Read the model definition and answer for the solid it produces. Units are mm, in the model's axes. Coordinates: 2 decimals unless noted, no trailing zeros. Order: outer loops, then holes, each group sorted by start corner. A loop starts at its lowest first (then second) coordinate and runs counter-clockwise, first axis right, second up.
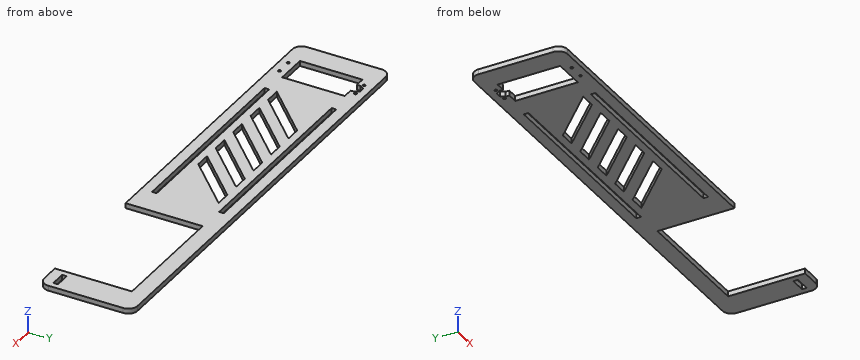
Autodesk Inventor part; units mm, degrees
ref_plane "YZ Plane" through (0, 0, 0) normal (1, 0, 0) x (0, 1, 0)
ref_plane "XZ Plane" through (0, 0, 0) normal (0, 1, 0) x (-1, 0, 0)
ref_plane "XY Plane" through (0, 0, 0) normal (0, 0, 1) x (1, 0, 0)
sketch "Sketch7" plane through (0, 0, 0) normal (0, 0, 1) x (1, 0, 0)
  line L0 (296.3, 0) -> (296.3, 60.7)
  line L1 (296.3, 60.7) -> (0, 60.7)
  line L2 (0, 60.7) -> (0, 0)
  line L3 (50.3, 10) -> (179.25, 10)
  line L4 (179.25, 10) -> (179.25, 7)
  line L5 (179.25, 7) -> (50.3, 7)
  line L6 (50.3, 7) -> (50.3, 10)
  line L7 (15, 50.75) -> (35.3, 50.75)
  line L8 (35.3, 50.75) -> (35.3, 9.95)
  line L9 (35.3, 9.95) -> (15, 9.95)
  line L10 (15, 9.95) -> (15, 50.75)
  line L11 (50.3, 50.7) -> (179.25, 50.7)
  line L12 (179.25, 50.7) -> (179.25, 53.7)
  line L13 (179.25, 53.7) -> (50.3, 53.7)
  line L14 (50.3, 53.7) -> (50.3, 50.7)
  line L15 (0, 0) -> (197.25, 0)
  line L16 (197.25, 0) -> (197.25, 50.2)
  line L17 (197.25, 50.2) -> (278.3, 50.2)
  line L18 (278.3, 50.2) -> (278.3, 0)
  line L19 (278.3, 0) -> (296.3, 0)
  line L20 (282.3, 10) -> (292.3, 10)
  line L21 (292.3, 10) -> (292.3, 7)
  line L22 (292.3, 7) -> (282.3, 7)
  line L23 (282.3, 7) -> (282.3, 10)
  point P0 (50.3, 52.2)
  point P1 (50.3, 8.5)
  dimension "d154" = 128.95
  dimension "d159" = 3
  dimension "d161" = 40.8
  dimension "d162" = 20.3
  dimension "d163" = 15
  dimension "d168" = 7
  dimension "d224" = 40.7
  dimension "d225" = 15
  dimension "d232" = 60.7
  dimension "d233" = 7
  dimension "d234" = 18
  dimension "d235" = 81.05
  dimension "d236" = 9.95
  dimension "d237" = 10.5
  dimension "d239" = 18
  dimension "d240" = 4
  dimension "d247" = 10
extrude "Extrusion7" add sketch "Sketch7" along normal blind 3.3 contours L19 L18 L17 L16 L15 L2 L1 L0 | L20 L21 L22 L23
fillet "Fillet1" radius 6 4 edges at (0, 60.7, 1.65) (0, 0, 1.65) (296.3, 60.7, 1.65) (296.3, 0, 1.65)
sketch "Sketch9" plane through (0, 0, 3.3) normal (0, 0, 1) x (1, 0, 0)
  arc A0 (290.3, 0) -> (296.3, 6) centre (290.3, 6) ccw
  line L0 (296.3, 6) -> (296.3, 54.7)
  arc A1 (296.3, 54.7) -> (290.3, 60.7) centre (290.3, 54.7) ccw
  line L1 (290.3, 60.7) -> (6, 60.7)
  arc A2 (6, 60.7) -> (0, 54.7) centre (6, 54.7) ccw
  line L2 (0, 54.7) -> (0, 6)
  arc A3 (0, 6) -> (6, 0) centre (6, 6) ccw
  line L3 (35.3, 50.75) -> (35.3, 9.95)
  line L4 (35.3, 9.95) -> (15, 9.95)
  line L5 (15, 9.95) -> (15, 50.75)
  line L6 (15, 50.75) -> (35.3, 50.75)
  line L7 (50.3, 50.7) -> (50.3, 53.7)
  line L8 (50.3, 53.7) -> (179.25, 53.7)
  line L9 (179.25, 53.7) -> (179.25, 50.7)
  line L10 (179.25, 50.7) -> (50.3, 50.7)
  line L11 (179.25, 10) -> (179.25, 7)
  line L12 (179.25, 7) -> (50.3, 7)
  line L13 (50.3, 7) -> (50.3, 10)
  line L14 (50.3, 10) -> (179.25, 10)
  line L15 (50.3, 15) -> (81, 45.7)
  line L16 (81, 45.7) -> (91, 45.7)
  line L17 (91, 45.7) -> (60.3, 15)
  line L18 (60.3, 15) -> (50.3, 15)
  line L19 (6, 0) -> (197.25, 0)
  line L20 (197.25, 0) -> (197.25, 50.2)
  line L21 (197.25, 50.2) -> (278.3, 50.2)
  line L22 (278.3, 50.2) -> (278.3, 0)
  line L23 (278.3, 0) -> (290.3, 0)
  point P0 (0, 0)
  dimension "d172" = 45
  dimension "d173" = 10
  dimension "d175" = 5
  dimension "d182" = 5
extrude "Extrusion8" cut sketch "Sketch9" against normal blind 3.3 contours L15 L16 L17 L18
sketch "Sketch10" plane through (0, 0, 3.3) normal (0, 0, 1) x (1, 0, 0)
  line L0 (15, 9.95) -> (15, 50.75)
  line L1 (15, 50.75) -> (35.3, 50.75)
  line L2 (35.3, 50.75) -> (35.3, 9.95)
  line L3 (35.3, 9.95) -> (15, 9.95)
  circle A0 centre (20, 54.7) radius 0.85
  circle A1 centre (30, 54.7) radius 0.85
  circle A2 centre (20, 5.2) radius 0.85
  circle A3 centre (30, 5.2) radius 0.85
  point P0 (0, 0)
  dimension "d183" = 1.7
  dimension "d184" = 5
  dimension "d185" = 10
  dimension "d186" = 5
  dimension "d187" = 10
  dimension "d188" = 3.95
  dimension "d189" = 4.75
extrude "Extrusion9" cut sketch "Sketch10" against normal blind 10 contours A0 | A1 | A2 | A3
sketch "Sketch11" plane through (0, 0, 3.3) normal (0, 0, 1) x (1, 0, 0)
  line L0 (15, 50.75) -> (35.3, 50.75)
  line L1 (21.4, 55.85) -> (28.6, 55.85) construction
  line L2 (28.6, 55.85) -> (28.6, 50.75) construction
  line L3 (28.6, 50.75) -> (21.4, 50.75)
  line L4 (21.4, 50.75) -> (21.4, 55.85) construction
  line L5 (15, 9.95) -> (15, 50.75)
  line L6 (35.3, 50.75) -> (35.3, 9.95)
  line L7 (259.7, 10) -> (259.7, 50.8)
  line L8 (21.4, 53.25) -> (23.2205, 55.85)
  line L9 (26.7795, 55.85) -> (28.6, 53.25)
  line L10 (21.4, 50.75) -> (21.4, 53.25)
  line L11 (23.2205, 55.85) -> (26.7795, 55.85)
  line L12 (28.6, 53.25) -> (28.6, 50.75)
  point P0 (0, 0)
  dimension "d203" = 6.4
  dimension "d205" = 5.1
  dimension "d206" = 7.2
  dimension "d215" = 35
  dimension "d216" = 2.5
  dimension "d217" = 35
extrude "Extrusion10" cut sketch "Sketch11" against normal blind 10
sketch "Sketch13" plane through (0, 0, 3.3) normal (0, 0, 1) x (1, 0, 0)
  line L0 (282.3, 10) -> (292.3, 10)
  line L1 (292.3, 10) -> (292.3, 7)
  line L2 (292.3, 7) -> (282.3, 7)
  line L3 (282.3, 7) -> (282.3, 10)
  point P0 (0, 0)
extrude "Extrusion11" cut sketch "Sketch13" against normal up to surface (3.3 mm away)
pattern_linear "Rectangular Pattern2" count 5 spacing 20 along (1, 0, 0) of "Extrusion8"
equation "\"base_servo\" = 20"
equation "\"altura_servo\" = 40"
equation "\"agujero_servo\" = 2"
equation "\"distancia_agujero_servo\" = 4.75"
equation "\"largo_base\" = 200"
properties part number "Cuerpo - LateralPrueba"
Q1. This flat-tipped pin is pushed along its axis until it touches: P1, Ø1.4, axis at x = 20, y = 5.2, coming from the +Z side. Where does it stop, or does it pass through?
Q2. The part is cut by section B-B, the plane y = 18. State how many separate pieces and enclosed holes the cut face has, then the cut area to 3 significant figures.
Q3. Straight lines are drawn through the part: L1, parallel to X at y = 11, z = 0.45; L2, parallel to Y at x = 30, z = 0.8; L3, parallel to Y at x = 139.5, z = 2.55. For each, find the intervals that lie inside material, in ascending order.
Q4. The part is cut by section D-D, the plane x = 237. Determine the outline of the cut face in (y, z), then the cut area to 4 significant figures.
Q5. The part is cut by section A-A, the plane x = 137. Determine the outline of the cut face in (y, z).
Computed values:
1. P1: passes through
2. separate pieces: 8
2. enclosed holes: 0
2. area: 478 mm2
3. L1: x = 0 to 15, 35.3 to 197.25, 278.3 to 296.3
3. L2: y = 0 to 4.35, 6.05 to 9.95, 50.75 to 53.85, 55.55 to 60.7
3. L3: y = 0 to 7, 10 to 15, 24.2 to 34.2, 44.2 to 50.7, 53.7 to 60.7
4. outline: (50.2, 0) - (60.7, 0) - (60.7, 3.3) - (50.2, 3.3) - close
4. area: 34.65 mm2
5. outline: (0, 0) - (7, 0) - (7, 3.3) - (0, 3.3) - close; (10, 0) - (15, 0) - (15, 3.3) - (10, 3.3) - close; (21.7, 0) - (31.7, 0) - (31.7, 3.3) - (21.7, 3.3) - close; (41.7, 0) - (50.7, 0) - (50.7, 3.3) - (41.7, 3.3) - close; (53.7, 0) - (60.7, 0) - (60.7, 3.3) - (53.7, 3.3) - close
